```python
from build123d import *

# Parameters (mm, degrees)
F0_W     = 38.1
F0_H     = 57.3024
F1_DEPTH = 12.7


with BuildPart() as f1:
    # F0 (on Front) → F1 (new body)
    with BuildSketch(Plane.XZ):
        with Locations((-19.05, 28.6512)):
            Rectangle(F0_W, F0_H)
        with BuildLine():
            ThreePointArc((-6.3221496252, 50.8), (-7.3520700194, 47.3248567906), (-10.1092, 44.972073202))
            Line((-10.1092, 44.972073202), (-10.1092, 31.1974352398))
            ThreePointArc((-10.1092, 31.1974352398), (-7.3720510513, 28.8547735092), (-6.35, 25.4))
            ThreePointArc((-6.35, 25.4), (-16.1547735092, 20.0720510513), (-15.2908, 31.1974352398))
            Line((-15.2908, 31.1974352398), (-15.2908, 44.972073202))
            ThreePointArc((-15.2908, 44.972073202), (-16.1751432094, 56.1479299806), (-6.3221496252, 50.8))
        make_face(mode=Mode.SUBTRACT)
        with BuildLine():
            ThreePointArc((-8.7376, 50.8), (-9.0967792407, 49.1515419569), (-10.1092, 47.8019391067))
            Line((-10.1092, 47.8019391067), (-10.1092, 44.972073202))
            ThreePointArc((-10.1092, 44.972073202), (-7.3520700194, 47.3248567906), (-6.3221496252, 50.8))
            ThreePointArc((-6.3221496252, 50.8), (-16.1751432094, 56.1479299806), (-15.2908, 44.972073202))
            Line((-15.2908, 44.972073202), (-15.2908, 47.8019391067))
            ThreePointArc((-15.2908, 47.8019391067), (-14.3484580431, 54.4032207593), (-8.7376, 50.8))
        make_face()
        with BuildLine():
            ThreePointArc((-15.2908, 50.8), (-12.7, 53.3908), (-10.1092, 50.8))
            Line((-10.1092, 50.8), (-10.1092, 47.8019391067))
            ThreePointArc((-10.1092, 47.8019391067), (-9.0967792407, 49.1515419569), (-8.7376, 50.8))
            ThreePointArc((-8.7376, 50.8), (-14.3484580431, 54.4032207593), (-15.2908, 47.8019391067))
            Line((-15.2908, 47.8019391067), (-15.2908, 50.8))
        make_face()
        with BuildLine():
            ThreePointArc((-8.7376, 25.4), (-9.0967792407, 27.0484580431), (-10.1092, 28.3980608933))
            Line((-10.1092, 28.3980608933), (-10.1092, 25.4))
            ThreePointArc((-10.1092, 25.4), (-12.7, 22.8092), (-15.2908, 25.4))
            Line((-15.2908, 25.4), (-15.2908, 28.3980608933))
            ThreePointArc((-15.2908, 28.3980608933), (-14.3484580431, 21.7967792407), (-8.7376, 25.4))
        make_face()
        with BuildLine():
            ThreePointArc((-6.35, 25.4), (-7.3720510513, 28.8547735092), (-10.1092, 31.1974352398))
            Line((-10.1092, 31.1974352398), (-10.1092, 28.3980608933))
            ThreePointArc((-10.1092, 28.3980608933), (-9.0967792407, 27.0484580431), (-8.7376, 25.4))
            ThreePointArc((-8.7376, 25.4), (-14.3484580431, 21.7967792407), (-15.2908, 28.3980608933))
            Line((-15.2908, 28.3980608933), (-15.2908, 31.1974352398))
            ThreePointArc((-15.2908, 31.1974352398), (-16.1547735092, 20.0720510513), (-6.35, 25.4))
        make_face()
        with Locations((19.05, 28.6512)):
            Rectangle(F0_W, F0_H)
        with BuildLine():
            Line((10.1092, 25.4), (10.1092, 50.8))
            ThreePointArc((10.1092, 50.8), (12.7, 53.3908), (15.2908, 50.8))
            Line((15.2908, 50.8), (15.2908, 25.4))
            ThreePointArc((15.2908, 25.4), (12.7, 22.8092), (10.1092, 25.4))
        make_face(mode=Mode.SUBTRACT)
    extrude(amount=F1_DEPTH)


solid = f1.part
```
Geometry check sheet. Reference: the model listing, model coordinates, mm. A direction names the side the tool comes from. Give positions to 0.01 mm unless a question says otherwise; leave off trailing zeros. Loops run counter-clockwise (first coordinate to the right, second up) from the corner with the lowest first, then second, coordinate; pieces in that order, holes last. Notation, with made-up numbers: M 76,37 L 81,37 A16 cw 81,66 Z; hole C 69.25,4.5 d2. An arc over 180 degrees is marked long. Write item = value, one per line.
(1) Release check for a two-part mould opening along X. For faces 1 (the face through (-1, 0, 29)), 2 (the face through (10.109, -6, 38)), 3 (the face through (38.1, -6, 28)) record: released by +X, released by -X, zero draft, split by the parting line, or undercut.
Answer below:
face_1 = zero draft
face_2 = undercut
face_3 = released by +X
(2) Sectioned sample at C-C, the plane x = 11.5. Record the cut outline in (y, z).
Answer below:
outline = M -12.7,0 L 0,0 L 0,23.1 L -12.7,23.1 Z; M -12.7,53.1 L 0,53.1 L 0,57.3 L -12.7,57.3 Z
(3) Sectioned sample at B-B, the plane y = -8. Record the cut outline in (x, z), plus the area to 3 significant figures.
Answer below:
outline = M -38.1,0 L 38.1,0 L 38.1,57.3 L -38.1,57.3 Z; hole M -15.29,25.4 A2.59 ccw -10.11,25.4 L -10.11,50.8 A2.59 ccw -15.29,50.8 Z; hole M 10.11,25.4 A2.59 ccw 15.29,25.4 L 15.29,50.8 A2.59 ccw 10.11,50.8 Z
area = 4,060 mm2
(4) Sectioned sample at A-A, the plane x = -12.7. Record the cut outline in (y, z), plus the area to 3 significant figures.
Answer below:
outline = M -12.7,0 L 0,0 L 0,22.81 L -12.7,22.81 Z; M -12.7,53.39 L 0,53.39 L 0,57.3 L -12.7,57.3 Z
area = 339 mm2
(5) Tool access check on faces 4 (the face through (1, -6, 57.302)), 5 (the face through (-12.64, -6.26, 22.81)). Record the directions out of +Z, -Z, +X, -X, +Y, -Y that give a thin tool (end or side, any length) a straight path to the whole face; none if there is none.
Answer below:
face_4 = +Z, +X, -X, +Y, -Y
face_5 = +Y, -Y
(6) Material ranges on line 1 (X direction, y = -10.25, z = 32); line 2 (Z direction, x = -12.5, y = -8.25); line 3 (Z direction, x = -13.5, y = -6), recorded low to high. Write a range as [from, to].
Answer below:
line_1 = [-38.1, -15.29], [-10.11, 10.11], [15.29, 38.1]
line_2 = [0, 22.82], [53.38, 57.3]
line_3 = [0, 22.94], [53.26, 57.3]
